CAD build for the part. Positions are in the model's coordinates, mm. Coordinates: 2 decimals unless noted, no trailing zeros. Order: outer loops, then holes, each group sorted by start corner. A loop starts at its lowest first (then second) coordinate and runs counter-clockwise, first axis right, second up. Notation, with made-up numbers: (7, 17.25) - (65, 17.25) arc R29 cw to (65, 41.25) - close; hole circle Ø3 at (0.5, 85.5). An arc over 180 degrees is marked (long way). Return JSON: item names as keys, results as strings.
from build123d import *

# Parameters (mm, degrees)
SKETCH1_W                  = 88.9
SKETCH1_H                  = 260.35
BOSS_EXTRUDE1_DEPTH        = 19.05
FILLET1_R                  = 3.175
F_3_8_0_3750_DOWEL_HOLE1_D = 9.525


with BuildPart() as part:
    # Sketch1 → Boss-Extrude1 (new, symmetric)
    with BuildSketch(Plane(origin=(0, 0, 0), x_dir=(0, 0, -1), z_dir=(1, 0, 0))):
        with Locations((44.45, 130.175)):
            Rectangle(SKETCH1_W, SKETCH1_H)
    extrude(amount=BOSS_EXTRUDE1_DEPTH, both=True)

    # Fillet1
    fillet1_edges = [part.edges().sort_by_distance(p)[0] for p in [
        (19.05, 130.175, 0),
        (-19.05, 130.175, 0),
        (-19.05, 130.175, -88.9),
        (19.05, 130.175, -88.9),
    ]]
    fillet(fillet1_edges, radius=FILLET1_R)

    # 3/8 (0.3750) Dowel Hole1 (through all)
    with Locations(Plane.ZY.offset(19.05)):
        with Locations((-44.45, 215.9), (-44.45, 44.45)):
            Hole(F_3_8_0_3750_DOWEL_HOLE1_D / 2)


solid = part.part
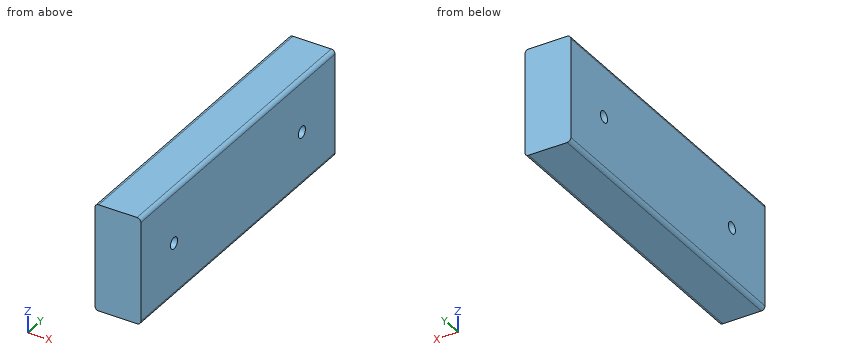
Item 1: Drop a flat-ended pin along its axis: P1, Ø7.5, axis at y = 44.45, z = -44.45, coming from the +X side. Give the stop position or say it passes through.
Findings below:
{"P1": "passes through"}
Item 2: Wall check: L1, parallel to Y at x = 3, z = -44.45; L2, parallel to Z at x = -10.5, y = 42.5; L3, parallel to Z at x = -16, y = 195. Give the ranges that are in metal, low to high. Write a range as [from, to].
Findings below:
{"L1": "y = [0, 39.69], [49.21, 211.14], [220.66, 260.35]", "L2": "z = [-88.9, -48.79], [-40.11, 0]", "L3": "z = [-88.9, 0]"}
Item 3: Band-saw the part on B-B, the plane z = -44.45. List the corners of the cut face in (x, y).
Findings below:
{"outline": "(-19.05, 0) - (19.05, 0) - (19.05, 39.69) - (-19.05, 39.69) - close; (-19.05, 49.21) - (19.05, 49.21) - (19.05, 211.14) - (-19.05, 211.14) - close; (-19.05, 220.66) - (19.05, 220.66) - (19.05, 260.35) - (-19.05, 260.35) - close"}
